For this review, take the finished solid that the model builds, in its own axes (mm). Coordinates: 2 decimals unless noted, no trailing zeros. Write each loop counter-clockwise with the first axis right and the second up, starting at its lowest first coordinate (ties: lowest second). Pieces come first, ordered by that corner, then holes. Notation, with made-up numbers: (47.5, 12.25) -> (66.5, 12.25) arc R32 cw to (66.5, 38.25) -> close; hole circle Ø4 at (-9.75, -2.75). An arc over 180 degrees is marked (long way). One line per item, written item: value. Start each with the question number.
1) For probe 1 along Y at (x, z) = (1.25, 125.5); probe 2 along Z at (x, y) = (-0.35, -96); probe 3 along Y at (x, z) = (0.3, -189.5), list the stretches that pass through material, from the lowest coordinate up. Write a range as from..to.
2) Add section B-B (y = -94). State the section outline as (x, z) points, and give its area (3 significant figures).
3) For pin 1 Ø1 at (x, z) = (-0.5, -227) entering from -Y, flat-tipped, find the tip position at first contact; note if it passes through.
4) Add section A-A (x = -0.7). State the section outline as (y, z) points.
5) Add section C-C (z = 185). State the section outline as (x, y) points, and give its area (3 significant figures).
from build123d import *

# Parameters (mm, degrees)
SKETCH1_W           = 498.348
SKETCH1_H           = 177.8
BOSS_EXTRUDE1_DEPTH = 1.5875
BOSS_EXTRUDE2_DEPTH = 3.175


with BuildPart() as part:
    # Sketch1 → Boss-Extrude1 (new, symmetric)
    with BuildSketch(Plane(origin=(0, 0, 0), x_dir=(0, 0, -1), z_dir=(1, 0, 0))):
        Rectangle(SKETCH1_W, SKETCH1_H)
    extrude(amount=BOSS_EXTRUDE1_DEPTH, both=True)

    # Sketch2 → Boss-Extrude2 (add)
    with BuildSketch(Plane(origin=(1.5875, 0, 0), x_dir=(0, 0, -1), z_dir=(1, 0, 0))):
        Polygon((249.174, -101.6), (249.174, -88.9), (48.2854, -88.9), (48.2854, -196.85), (149.8854, -196.85), (185.674, -101.6), align=None)
    extrude(amount=-BOSS_EXTRUDE2_DEPTH)


solid = part.part
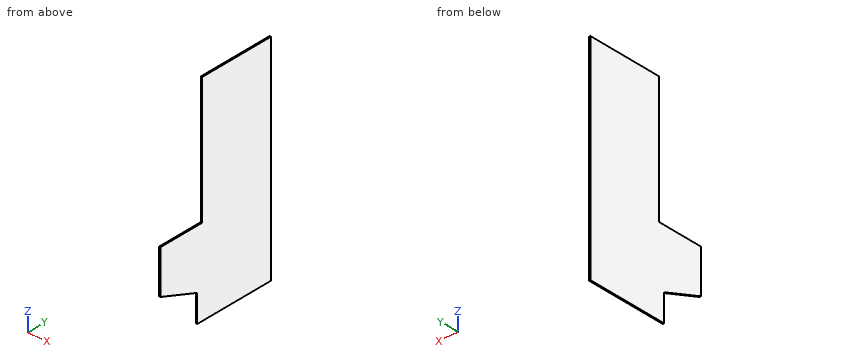
Numbers:
1. probe 1: -88.9..88.9
1. probe 2: -249.17..-48.29
1. probe 3: -101.6..88.9
2. outline: (-1.59, -249.17) -> (1.59, -249.17) -> (1.59, -48.29) -> (-1.59, -48.29) -> close
2. area: 638 mm²
3. pin 1: y = -101.6
4. outline: (-196.85, -149.89) -> (-101.6, -185.67) -> (-101.6, -249.17) -> (88.9, -249.17) -> (88.9, 249.17) -> (-88.9, 249.17) -> (-88.9, -48.29) -> (-196.85, -48.29) -> close
5. outline: (-1.59, -88.9) -> (1.59, -88.9) -> (1.59, 88.9) -> (-1.59, 88.9) -> close
5. area: 565 mm²
